Verification items for the finished model (mm, model axes). A direction names the side the tool comes from. Give positions to 0.01 mm unless a question says otherwise; leave off trailing zeros. Write each loop counter-clockwise with the first axis right and the second up, starting at its lowest first coordinate (ties: lowest second). Pieces come first, ordered by that corner, then holes. Notation, with made-up numbers: (3, 45.5) -> (60, 45.5) arc R23 cw to (60, 53.5) -> close; hole circle Ø9 at (42.5, -17.5). An arc over 180 degrees is marked (long way). Write item = value, one per line.
from build123d import *

# Parameters (mm, degrees)
SKETCH1_R           = 44.85
BOSS_EXTRUDE1_DEPTH = 15
SKETCH2_R           = 62.5
BOSS_EXTRUDE2_DEPTH = 10
SKETCH3_R           = 40
CUT_EXTRUDE1_DEPTH  = 15
SKETCH4_W           = 3.5
SKETCH4_H           = 3.5
SKETCH7_R           = 2.6
CUT_EXTRUDE4_DEPTH  = 92.855865354
CIRPATTERN1_COUNT   = 4
CUT_EXTRUDE6_DEPTH  = 10


with BuildPart() as part:
    # Sketch1 → Boss-Extrude1 (new body)
    with BuildSketch(Plane.XY):
        Circle(SKETCH1_R)
    extrude(amount=BOSS_EXTRUDE1_DEPTH)

    # Sketch2 → Boss-Extrude2 (add)
    with BuildSketch(Plane(origin=(0, 0, 0), x_dir=(-1, 0, 0), z_dir=(0, 0, -1))):
        Circle(SKETCH2_R)
    extrude(amount=BOSS_EXTRUDE2_DEPTH)

    # Sketch3 → Cut-Extrude1 (cut)
    with BuildSketch(Plane.XY.offset(15)):
        Circle(SKETCH3_R)
    extrude(amount=-CUT_EXTRUDE1_DEPTH, mode=Mode.SUBTRACT)

    # Sketch4 → Cut-Revolve1 (revolve, cut)
    with BuildSketch(Plane(origin=(0, 0, 0), x_dir=(0, 0, -1), z_dir=(1, 0, 0)), mode=Mode.PRIVATE) as cut_revolve1_sk:
        with Locations((-10.75, 44.3)):
            Rectangle(SKETCH4_W, SKETCH4_H)
        with Locations((-4.75, 44.3)):
            Rectangle(SKETCH4_W, SKETCH4_H)
    revolve(cut_revolve1_sk.sketch.rotate(Axis((0, 0, -42.713110189), (0, 0, 1)), 90), axis=Axis((0, 0, -42.713110189), (0, 0, 1)), mode=Mode.SUBTRACT)

    # Sketch7 → Cut-Extrude4 (cut, through all)
    with BuildSketch(Plane(origin=(0, 0, -10), x_dir=(-1, 0, 0), z_dir=(0, 0, -1))):
        with Locations((56.25, 0)):
            Circle(SKETCH7_R)
    cut_extrude4 = extrude(amount=-CUT_EXTRUDE4_DEPTH, mode=Mode.SUBTRACT)

    # CirPattern1: Cut-Extrude4 ×4 about axis
    cirpattern1_axis = Axis((0, 0, 0), (0, 0, 1))
    for i in range(1, CIRPATTERN1_COUNT):
        add(cut_extrude4.rotate(cirpattern1_axis, i * 360 / CIRPATTERN1_COUNT), mode=Mode.SUBTRACT)

    # Sketch9 → Cut-Extrude6 (cut)
    with BuildSketch(Plane.XY):
        with BuildLine():
            add(Edge.make_bspline(
                [(-0.55461157, -62.4975392), (-8.100511472, -62.208727423), (-7.033582927, -51.397803822), (-13.070361778, -48.779254228)],
                knots=[0.023286113, 0.023286113, 0.023286113, 0.023286113, 1, 1, 1, 1], degree=3))
            ThreePointArc((-13.070361778, -48.779254228), (-35.70889245, -35.70889245), (-48.779254228, -13.070361778))
            add(Edge.make_bspline(
                [(-62.4975392, -0.55461157), (-62.208727423, -8.100511472), (-51.397803822, -7.033582927), (-48.779254228, -13.070361778)],
                knots=[0.023286113, 0.023286113, 0.023286113, 0.023286113, 1, 1, 1, 1], degree=3))
            ThreePointArc((-62.4975392, -0.55461157), (-44.194173824, -44.194173824), (-0.55461157, -62.4975392))
        make_face()
        with BuildLine():
            ThreePointArc((-48.779254228, 13.070361778), (-35.70889245, 35.70889245), (-13.070361778, 48.779254228))
            add(Edge.make_bspline(
                [(-0.55461157, 62.4975392), (-8.100511472, 62.208727423), (-7.033582927, 51.397803822), (-13.070361778, 48.779254228)],
                knots=[0.023286113, 0.023286113, 0.023286113, 0.023286113, 1, 1, 1, 1], degree=3))
            ThreePointArc((-0.55461157, 62.4975392), (-44.194173824, 44.194173824), (-62.4975392, 0.55461157))
            add(Edge.make_bspline(
                [(-62.4975392, 0.55461157), (-62.208727423, 8.100511472), (-51.397803822, 7.033582927), (-48.779254228, 13.070361778)],
                knots=[0.023286113, 0.023286113, 0.023286113, 0.023286113, 1, 1, 1, 1], degree=3))
        make_face()
        with BuildLine():
            add(Edge.make_bspline(
                [(62.498616294, -0.415886171), (62.283969661, -8.150798689), (51.453042115, -6.968928103), (48.779254228, -13.070361778)],
                knots=[0.017259954, 0.017259954, 0.017259954, 0.017259954, 1, 1, 1, 1], degree=3))
            ThreePointArc((48.779254228, -13.070361778), (35.70889245, -35.70889245), (13.070361778, -48.779254228))
            add(Edge.make_bspline(
                [(0.55461157, -62.4975392), (8.100511472, -62.208727423), (7.033582927, -51.397803822), (13.070361778, -48.779254228)],
                knots=[0.023286113, 0.023286113, 0.023286113, 0.023286113, 1, 1, 1, 1], degree=3))
            ThreePointArc((0.55461157, -62.4975392), (44.24319492, -44.145098293), (62.498616294, -0.415886171))
        make_face()
        with BuildLine():
            ThreePointArc((13.070361778, 48.779254228), (35.70889245, 35.70889245), (48.779254228, 13.070361778))
            add(Edge.make_bspline(
                [(62.498616294, 0.415886171), (62.283969661, 8.150798689), (51.453042115, 6.968928103), (48.779254228, 13.070361778)],
                knots=[0.017259954, 0.017259954, 0.017259954, 0.017259954, 1, 1, 1, 1], degree=3))
            ThreePointArc((62.498616294, 0.415886171), (44.24319492, 44.145098293), (0.55461157, 62.4975392))
            add(Edge.make_bspline(
                [(0.55461157, 62.4975392), (8.100511472, 62.208727423), (7.033582927, 51.397803822), (13.070361778, 48.779254228)],
                knots=[0.023286113, 0.023286113, 0.023286113, 0.023286113, 1, 1, 1, 1], degree=3))
        make_face()
    extrude(amount=-CUT_EXTRUDE6_DEPTH, mode=Mode.SUBTRACT)


solid = part.part
Item 1: Sectioned sample at B-B on z = -3. Give the number of separate pieces and of enclosed holes in the cut face, then the cut area to 3 significant figures.
Response values:
separate_pieces = 1
enclosed_holes = 4
area = 8,650 mm^2
Item 2: Sectioned sample at C-C on x = 23. Record the cut outline in (y, z).
Response values:
outline = (-44.96, -10) -> (44.96, -10) -> (44.96, 0) -> (38.5, 0) -> (38.5, 3) -> (35.8, 3) -> (35.8, 6.5) -> (38.5, 6.5) -> (38.5, 9) -> (35.8, 9) -> (35.8, 12.5) -> (38.5, 12.5) -> (38.5, 15) -> (32.73, 15) -> (32.73, 0) -> (-32.73, 0) -> (-32.73, 15) -> (-38.5, 15) -> (-38.5, 12.5) -> (-35.8, 12.5) -> (-35.8, 9) -> (-38.5, 9) -> (-38.5, 6.5) -> (-35.8, 6.5) -> (-35.8, 3) -> (-38.5, 3) -> (-38.5, 0) -> (-44.96, 0) -> close
Item 3: Sectioned sample at A-A on y = 29. Record the cut outline in (x, z), then the cut area to 3 significant figures.
Response values:
outline = (-41.34, -10) -> (41.34, -10) -> (41.34, 0) -> (34.21, 0) -> (34.21, 3) -> (31.14, 3) -> (31.14, 6.5) -> (34.21, 6.5) -> (34.21, 9) -> (31.14, 9) -> (31.14, 12.5) -> (34.21, 12.5) -> (34.21, 15) -> (27.55, 15) -> (27.55, 0) -> (-27.55, 0) -> (-27.55, 15) -> (-34.21, 15) -> (-34.21, 12.5) -> (-31.14, 12.5) -> (-31.14, 9) -> (-34.21, 9) -> (-34.21, 6.5) -> (-31.14, 6.5) -> (-31.14, 3) -> (-34.21, 3) -> (-34.21, 0) -> (-41.34, 0) -> close
area = 984 mm^2
Item 4: Go/stop test with flat-tipped pins: P1, Ø8, axis at x = 10, z = 12, coming from the -Y side; P2, Ø4.5, axis at x = 0, y = -56.25, coming from the -Z side; P3, Ø7, axis at x = -56.25, y = 0, coming from the +Z side; P4, Ø6, axis at x = 4, z = -5, coming from the +Y side. Record where each tip stops, or that it passes through.
Response values:
P1 = -44.44
P2 = through
P3 = 0
P4 = 62.47
Item 5: Mould release check, pull along Y, two halves, no side actions. Record for faces 1 (the flat face through (-1, 1, 0)), 2 (the cylindrical face through (-35.59, -27.29, 7.73)), 3 (the flat face through (40, 16, 3)): +Y half, -Y half, draft (parallel to the pull), parting line (faces both ways), or undercut.
Response values:
face_1 = undercut
face_2 = parting line
face_3 = draft
Item 6: Material ranges on line 1 (Z direction, x = 42, y = -14); line 2 (Y direction, x = 11, z = 1.5); line 3 (X direction, y = -56.25, z = -7.5), recorded low to high.
Response values:
line_1 = -10 to 3, 6.5 to 9, 12.5 to 15
line_2 = -43.48 to -38.46, 38.46 to 43.48
line_3 = -7.5 to -2.6, 2.6 to 7.5
Item 7: Set-up check for faces 4 (the cylindrical face through (53.653, -0.114, -5.07)), 5 (the cylindrical face through (33.766, 25.891, 10.726)), 6 (the cylindrical face through (-35.59, -27.29, 13.73)): record each of +Z, -Z, +X, -X, +Y, -Y from which the full face is reachable in a straight line by a thin tool's end or side.
Response values:
face_4 = +Z, -Z
face_5 = none
face_6 = +Z
